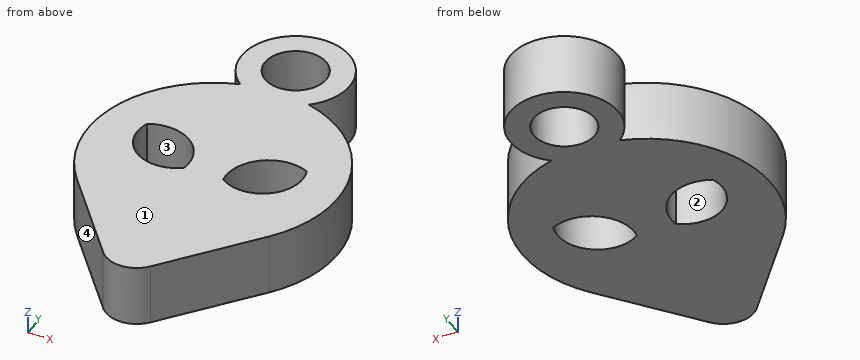
from build123d import *

# Parameters (mm, degrees)
F1_DEPTH = 12.7
F2_R     = 6.325984
F3_DEPTH = 12.7


with BuildPart() as f1:
    # F0 (on Top) → F1 (new body)
    with BuildSketch(Plane.XY):
        with BuildLine():
            Line((4.930796, -34.827771), (20.013764, -16.240678))
            ThreePointArc((20.013764, -16.240678), (0, 25.774219), (-20.013764, -16.240678))
            Line((-20.013764, -16.240678), (-4.930796, -34.827771))
            ThreePointArc((-4.930796, -34.827771), (0, -37.176552), (4.930796, -34.827771))
        make_face()
        with BuildLine():
            ThreePointArc((-16.655875, 5.560721), (-7.460285, 4.715734), (-4.074331, -3.875436))
            ThreePointArc((-4.074331, -3.875436), (-13.849756, -3.803562), (-16.655875, 5.560721))
        make_face(mode=Mode.SUBTRACT)
        with BuildLine():
            ThreePointArc((16.655875, 5.560721), (13.849756, -3.803562), (4.074331, -3.875436))
            ThreePointArc((4.074331, -3.875436), (7.460285, 4.715734), (16.655875, 5.560721))
        make_face(mode=Mode.SUBTRACT)
    extrude(amount=F1_DEPTH)

    # F2 (on face) → F3 (join)
    with BuildSketch(Plane(origin=(0, 0, 0), x_dir=(1, 0, 0), z_dir=(0, 0, -1))):
        with BuildLine():
            ThreePointArc((7.156011, -24.760894), (0, -25.774219), (-7.156011, -24.760894))
            ThreePointArc((-7.156011, -24.760894), (0, -44.494381), (7.156011, -24.760894))
        make_face()
        with Locations((0, -33.330135)):
            Circle(F2_R, mode=Mode.SUBTRACT)
    extrude(amount=-F3_DEPTH)


solid = f1.part
Check sheet for the modelled part. Datum: model origin and axes. Units: mm. Face numbers are marked on the shaded views. Give positions to 0.01 mm unless a question says otherwise; leave off trailing zeros. Loops run counter-clockwise (first coordinate to the right, second up) from the corner with the lowest first, then second, coordinate; pieces in that order, holes last. Notation, with made-up numbers: M 35.5,28 L 67.5,28 A14 ccw 67.5,55 Z; hole C -28.75,74.25 d7. An arc over 180 degrees is marked long. Return JSON: item names as keys, results as strings. Group by question number.
1. Cross-section at A-A on x = 0. Record the boundary of the cut face in (y, z).
2. Cross-section at D-D on y = 19. Record the boundary of the cut face in (x, z), plus the area to 3 significant figures.
3. Go/stop test with flat-tipped pins: pin 1 (1.5 mm diameter, centred on x = -13, z = 7.5, fed in from -Y); pin 2 (10 mm diameter, centred on x = 0, y = 33.33, fed in from -Z); pin 3 (5 mm diameter, centred on x = -16, z = 3, fed in from +Y); pin 4 (6 mm diameter, centred on y = 35.5, z = 8, fed in from -X). Record where each tip stops, or that it passes through.
4. Cross-section at B-B on y = 37. Record the boundary of the cut face in (x, z).
5. Thickness scan on L1, parallel to Y at x = 10, z = 10.25; L2, parallel to Y at x = 0.5, z = 11.25; L3, parallel to X at y = 35, z = 1.75. Record the ranges inside material, lowest first.
6. Cross-section at C-C on z = 8.5. Record the boundary of the cut face in (x, y).
7. Mould release check, pull along Y, two halves, no side actions. Record for the marked faces 1, 2, 3 and 4: released by +Y, released by -Y, zero draft, split by the parting line, or undercut.
Return value:
{
 "1": {"outline": "M -37.18,0 L 27,0 L 27,12.7 L -37.18,12.7 Z; M 39.66,0 L 44.49,0 L 44.49,12.7 L 39.66,12.7 Z"},
 "2": {"outline": "M -17.42,0 L 17.42,0 L 17.42,12.7 L -17.42,12.7 Z", "area": "442 mm^2"},
 "3": {"pin 1": "y = -25.81", "pin 2": "through", "pin 3": "y = 21.96", "pin 4": "x = -11.16"},
 "4": {"outline": "M -10.54,0 L -5.15,0 L -5.15,12.7 L -10.54,12.7 Z; M 5.15,0 L 10.54,0 L 10.54,12.7 L 5.15,12.7 Z"},
 "5": {"L1": "-28.58 to -5.38, 6.04 to 23.76, 28.37 to 38.29", "L2": "-37.16 to 27.02, 39.64 to 44.48", "L3": "-11.04 to -6.1, 6.1 to 11.04"},
 "6": {"outline": "M -20.01,-16.24 L -4.93,-34.83 A6.35 ccw 4.93,-34.83 L 20.01,-16.24 A25.77 ccw 7.16,24.76 A11.16 ccw long -7.16,24.76 A25.77 ccw Z; hole M -16.66,5.56 A8.23 ccw -4.07,-3.88 A8.81 ccw Z; hole C 0,33.33 d12.65; hole M 4.07,-3.88 A8.23 ccw 16.66,5.56 A8.81 ccw Z"},
 "7": {"face 1": "zero draft", "face 2": "undercut", "face 3": "undercut", "face 4": "released by -Y"}
}
